Source: CAD feature listing. Evaluate the final solid. Frame: model axes, mm. Face numbers are marked on the shaded views. A direction names the side the tool comes from. Give positions to 0.01 mm unless a question says otherwise; leave off trailing zeros. Return JSON: item names as keys, results as strings. Group by question number.
(1) Ray query, line 1 (X direction, y = -37.5, z = -13); line 2 (Z direction, x = 70, y = -31); line 3 (X direction, y = -8.5, z = -28.5). Return the intervals inside material, ascending. Write a range as from..to.
(2) Draft query along Y for the marked faces 1, 2 and 3. Return one class per face: released by +Y, released by -Y, zero draft, split by the parting line, or undercut.
(3) Access query for the marked faces 4 and 5. Directions: +Z, -Z, +X, -X, +Y, -Y. A direction counts if a zero-diameter tool reaches every point of the face in a straight line with its end or side. Return the directions, or none.
(4) Pin query (flat end, axial travel): pin 1 (3 mm diameter, centred on y = -28.5, z = 9.5, fed in from -X); pin 2 (2 mm diameter, centred on x = -72.5, y = -33.5, fed in from +Z). Return the tip coordinate at first contact, or that it passes through.
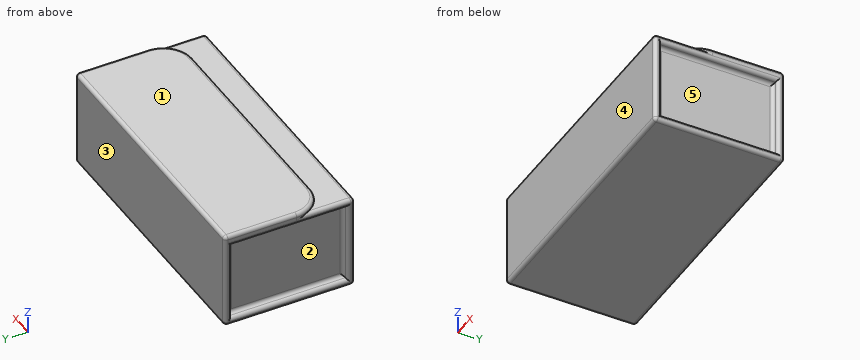
```python
from build123d import *

# Parameters (mm, degrees)
SKETCH_1_W          = 190
SKETCH_1_H          = 65
EXTRUDE_1_DEPTH     = 45
SKETCH_3_W          = 55
SKETCH_3_H          = 80
CUT_EXTRUDE_1_DEPTH = 5
EXTRUDE_2_DEPTH     = 2.5
FILLET_2_R          = 2.5
FILLET_3_R          = 2.5
FILLET_4_R          = 2.5


# Some blends are built 0.0001 mm under size
with BuildPart() as part:
    # ｽｹｯﾁ1 → ﾎﾞｽ - 押し出し1 (new, symmetric)
    with BuildSketch(Plane(origin=(0, 0, 0), x_dir=(1, 0, 0), z_dir=(0, 1, 0))):
        Rectangle(SKETCH_1_W, SKETCH_1_H)
    extrude(amount=EXTRUDE_1_DEPTH, both=True)

    # ｽｹｯﾁ3 → ｶｯﾄ - 押し出し1 (cut)
    with BuildSketch(Plane(origin=(95, 0, 0), x_dir=(0, 0, -1), z_dir=(1, 0, 0))):
        Rectangle(SKETCH_3_W, SKETCH_3_H)
    cut_extrude_1 = extrude(amount=-CUT_EXTRUDE_1_DEPTH, mode=Mode.SUBTRACT)

    # ﾐﾗｰ1: ｶｯﾄ - 押し出し1 across plane
    add(cut_extrude_1.mirror(Plane(origin=(0, 0, 0), x_dir=(0, 0, 1), z_dir=(1, 0, 0))), mode=Mode.SUBTRACT)

    # ｽｹｯﾁ4 → ﾎﾞｽ - 押し出し2 (add)
    with BuildSketch(Plane.XY.offset(32.5)):
        with BuildLine():
            Line((-95, 45), (95, 45))
            Line((95, 45), (95, -5))
            ThreePointArc((95, -5), (89.142135624, -19.142135624), (75, -25))
            Line((75, -25), (-75, -25))
            ThreePointArc((-75, -25), (-89.142135624, -19.142135624), (-95, -5))
            Line((-95, -5), (-95, 45))
        make_face()
    extrude(amount=EXTRUDE_2_DEPTH)

    # ﾌｨﾚｯﾄ2
    fillet_2_edges = [part.edges().sort_by_distance(p)[0] for p in [
        (0, -45, -32.5),
        (-95, -45, 0),
        (0, -45, 32.5),
        (95, -45, 0),
        (-90, -40, 0),
        (-90, 0, -27.5),
        (-90, 40, 0),
        (-90, 0, 27.5),
        (90, 40, 0),
        (90, 0, -27.5),
        (90, -40, 0),
        (90, 0, 27.5),
        (95, -25, 32.5),
        (95, 0, -32.5),
        (95, 45, 1.25),
        (95, 0, 27.5),
        (95, -40, 0),
        (95, 0, -27.5),
        (95, 40, 0),
        (-95, -25, 32.5),
        (-95, 0, -32.5),
        (-95, 45, 1.25),
        (-95, 0, -27.5),
        (-95, -40, 0),
        (-95, 0, 27.5),
        (-95, 40, 0),
    ]]
    fillet(fillet_2_edges, radius=FILLET_2_R - 0.0001)  # a hair under: the kernel refuses the full size

    # ﾌｨﾚｯﾄ3
    fillet_3_edges = [part.edges().sort_by_distance(p)[0] for p in [
        (94.267796242, 44.267796242, 35),
        (95, 18.75005, 35),
        (89.142135624, -19.142135624, 35),
        (0, -25, 35),
        (-89.142135624, -19.142135624, 35),
        (-95, 18.75005, 35),
        (-94.267796242, 44.267796242, 35),
        (0, 45, 35),
    ]]
    fillet(fillet_3_edges, radius=FILLET_3_R - 0.0001)  # a hair under: the kernel refuses the full size

    # ﾌｨﾚｯﾄ4
    # the kernel refuses this fillet: 2.5 mm, written as the material it takes off along each edge
    with BuildSketch(Plane(origin=(95, 42.5, -30), x_dir=(0, 0, -1), z_dir=(0, -1, 0))) as fillet_4_piece_1:
        with BuildLine():
            CenterArc((0.0001, -2.4999), 2.4999, 0, 90)
            Line((2.5, -2.4999), (2.5, 0))
            Line((2.5, 0), (0.0001, 0))
        make_face()
    revolve(axis=Axis((95, 42.5, -30), (1, 0, 0)), revolution_arc=90, mode=Mode.SUBTRACT)
    with BuildSketch(Plane(origin=(-95, 42.5, -30), x_dir=(0, 1, 0), z_dir=(0, 0, 1))) as fillet_4_piece_2:
        with BuildLine():
            CenterArc((0.0001, -2.4999), 2.4999, 0, 90)
            Line((2.5, -2.4999), (2.5, 0))
            Line((2.5, 0), (0.0001, 0))
        make_face()
    revolve(axis=Axis((-95, 42.5, -30), (-1, 0, 0)), revolution_arc=90, mode=Mode.SUBTRACT)
    with BuildSketch(Plane(origin=(95, 45, -32.5), x_dir=(0, 0, 1), z_dir=(-1, 0, 0))) as fillet_4_piece_3:
        with BuildLine():
            CenterArc((FILLET_4_R, -FILLET_4_R), FILLET_4_R, 90, 90)
            Line((0, -FILLET_4_R), (0, 0))
            Line((0, 0), (FILLET_4_R, 0))
        make_face()
    extrude(amount=190, mode=Mode.SUBTRACT)


solid = part.part
```
Answers:
{
 "1": {"line 1": "-90..90", "line 2": "-32.5..32.5", "line 3": "-94.5..94.5"},
 "2": {"face 1": "zero draft", "face 2": "undercut", "face 3": "released by +Y"},
 "3": {"face 4": "+Z, -Z, +X, -X, -Y", "face 5": "+X"},
 "4": {"pin 1": "x = -90", "pin 2": "z = 32.5"}
}
